Work out the finished part from the listing and answer in its coordinate system (mm). A direction names the side the tool comes from. Coordinates: 2 decimals unless noted, no trailing zeros. Loops run counter-clockwise (first coordinate to the right, second up) from the corner with the lowest first, then second, coordinate; pieces in that order, holes last. Notation, with made-up numbers: (-13, 39.25) -> (42, 39.25) arc R27 ccw to (42, 78.25) -> close; hole circle Ø8 at (51, 86.25). An arc over 180 degrees is marked (long way). Answer as CSV lines item,"result".
```python
from build123d import *

# Parameters (mm, degrees)
SKIZZE2_W                            = 100
SKIZZE2_H                            = 39.364160046
AUFSATZ_LINEAR_AUSTRAGEN1_DEPTH      = 30
SCHNITT_LINEAR_AUSTRAGEN1_DEPTH      = 40
SCHNITT_LINEAR_AUSTRAGEN1_DEPTH_BACK = 40
SKIZZE10_R                           = 5
SKIZZE17_R                           = 1.55
SCHNITT_LINEAR_AUSTRAGEN2_DEPTH      = 3
SKIZZE24_R                           = 1.55
SCHNITT_LINEAR_AUSTRAGEN4_DEPTH      = 112.577493681
SKIZZE37_R                           = 0.736865544
SCHNITT_LINEAR_AUSTRAGEN9_DEPTH      = 112.577493681
SKIZZE40_R                           = 2.1
SCHNITT_LINEAR_AUSTRAGEN10_DEPTH     = 6
SKIZZE42_R                           = 0.75
SCHNITT_LINEAR_AUSTRAGEN12_DEPTH     = 10
SKIZZE46_R                           = 2.85
SCHNITT_LINEAR_AUSTRAGEN15_DEPTH     = 10
SCHNITT_LINEAR_START                 = -5
SCHNITT_LINEAR_AUSTRAGEN25_DEPTH     = 2.7
LINEARES_MUSTER1_COUNT               = 5
LINEARES_MUSTER1_PITCH               = 17
SPIEGELN2_COPY_1_SKETCH_R            = 2.85
SPIEGELN2_COPY_1_DEPTH               = 10
SPIEGELN2_COPY_2_SKETCH_R            = 2.85
SPIEGELN2_COPY_2_DEPTH               = 10
SPIEGELN2_COPY_3_SKETCH_R            = 2.85
SPIEGELN2_COPY_3_DEPTH               = 10
SPIEGELN2_COPY_4_SKETCH_R            = 2.85
SPIEGELN2_COPY_4_DEPTH               = 10
SPIEGELN2_START                      = -5
SPIEGELN2_COPY_5_DEPTH               = 2.7
SPIEGELN2_COPY_6_DEPTH               = 2.7
SPIEGELN2_COPY_7_DEPTH               = 2.7
SPIEGELN2_COPY_8_DEPTH               = 2.7
SKIZZE51_R                           = 1.55
SCHNITT_LINEAR_AUSTRAGEN26_DEPTH     = 112.577493681
SKIZZE55_R                           = 0.5
SCHNITT_LINEAR_AUSTRAGEN28_DEPTH     = 112.577493681
SKIZZE59_R                           = 2.05
SCHNITT_LINEAR_AUSTRAGEN30_DEPTH     = 5
FASE1_SIZE                           = 1
FASE2_SIZE                           = 1
ABSPALTEN3_SURFACE_1_BACK            = 112.577
ABSPALTEN3_SURFACE_1_DEPTH           = 225.154


with BuildPart() as part:
    # Skizze2 → Aufsatz-Linear austragen1 (new body)
    with BuildSketch(Plane.XY):
        with Locations((50, 19.682080023)):
            Rectangle(SKIZZE2_W, SKIZZE2_H)
    extrude(amount=AUFSATZ_LINEAR_AUSTRAGEN1_DEPTH)

    # Skizze10 → Schnitt-Linear austragen1 (cut, two sides: drawn at the far end of the back side and taken through both)
    with BuildSketch(Plane.ZY.offset(-50).offset(-SCHNITT_LINEAR_AUSTRAGEN1_DEPTH_BACK)):
        with Locations((14.945770016, 20.027045739)):
            Circle(SKIZZE10_R)
    extrude(amount=SCHNITT_LINEAR_AUSTRAGEN1_DEPTH + SCHNITT_LINEAR_AUSTRAGEN1_DEPTH_BACK, mode=Mode.SUBTRACT)

    # Skizze17 → Schnitt-Linear austragen2 (cut)
    with BuildSketch(Plane.ZY.offset(-90)):
        with Locations((14.945770016, 20.027045739)):
            Circle(SKIZZE17_R)
    schnitt_linear_austragen2 = extrude(amount=-SCHNITT_LINEAR_AUSTRAGEN2_DEPTH, mode=Mode.SUBTRACT)

    # Spiegeln1: Schnitt-Linear austragen2 across plane
    add(schnitt_linear_austragen2.mirror(Plane.ZY.offset(-50)), mode=Mode.SUBTRACT)

    # Skizze24 → Schnitt-Linear austragen4 (cut, through all)
    with BuildSketch(Plane.XY.offset(30)):
        with Locations((16, 31.364160046)):
            Circle(SKIZZE24_R)
        with Locations((33, 31.364160046)):
            Circle(SKIZZE24_R)
        with Locations((50, 31.364160046)):
            Circle(SKIZZE24_R)
        with Locations((67, 31.364160046)):
            Circle(SKIZZE24_R)
        with Locations((84, 31.364160046)):
            Circle(SKIZZE24_R)
    schnitt_linear_austragen4 = extrude(amount=-SCHNITT_LINEAR_AUSTRAGEN4_DEPTH, mode=Mode.SUBTRACT)

    # Skizze37 → Schnitt-Linear austragen9 (cut, through all)
    with BuildSketch(Plane(origin=(100, 0, 0), x_dir=(0, 0, -1), z_dir=(1, 0, 0))):
        with Locations((-18.924590299, 18.633559666)):
            Circle(SKIZZE37_R)
    extrude(amount=-SCHNITT_LINEAR_AUSTRAGEN9_DEPTH, mode=Mode.SUBTRACT)

    # Skizze40 → Schnitt-Linear austragen10 (cut)
    with BuildSketch(Plane(origin=(100, 0, 0), x_dir=(0, 0, -1), z_dir=(1, 0, 0))):
        with Locations((-18.924590299, 18.633559666)):
            Circle(SKIZZE40_R)
    extrude(amount=-SCHNITT_LINEAR_AUSTRAGEN10_DEPTH, mode=Mode.SUBTRACT)

    # Skizze42 → Schnitt-Linear austragen12 (cut)
    with BuildSketch(Plane.ZY):
        with Locations((10.86415918, 18.842582577)):
            Circle(SKIZZE42_R)
    extrude(amount=-SCHNITT_LINEAR_AUSTRAGEN12_DEPTH, mode=Mode.SUBTRACT)

    # Skizze46 → Schnitt-Linear austragen15 (cut)
    with BuildSketch(Plane(origin=(0, 0, 0), x_dir=(-1, 0, 0), z_dir=(0, 0, -1))):
        with Locations((-84, 31.364160046)):
            Circle(SKIZZE46_R)
    schnitt_linear_austragen15 = extrude(amount=-SCHNITT_LINEAR_AUSTRAGEN15_DEPTH, mode=Mode.SUBTRACT)

    # Skizze50 → Schnitt-Linear austragen25 (cut)
    with BuildSketch(Plane.XY.offset(30).offset(SCHNITT_LINEAR_START)):
        Polygon((81.15, 33.009608314), (81.15, 39.364160046), (86.85, 39.364160046), (86.85, 33.009608314), (86.85, 29.718711779), (84, 28.073263512), (81.15, 29.718711779), align=None)
    schnitt_linear_austragen25 = extrude(amount=-SCHNITT_LINEAR_AUSTRAGEN25_DEPTH, mode=Mode.SUBTRACT)

    # Lineares Muster1: Schnitt-Linear austragen15, Schnitt-Linear austragen25 ×5
    with Locations(*[(-i * LINEARES_MUSTER1_PITCH, 0, 0) for i in range(1, LINEARES_MUSTER1_COUNT)]):
        add(schnitt_linear_austragen15, mode=Mode.SUBTRACT)
        add(schnitt_linear_austragen25, mode=Mode.SUBTRACT)

    # Spiegeln2: Schnitt-Linear austragen15, Schnitt-Linear austragen25 across plane
    add(schnitt_linear_austragen15.mirror(Plane.ZX.offset(19.764160046)), mode=Mode.SUBTRACT)
    add(schnitt_linear_austragen25.mirror(Plane.ZX.offset(19.764160046)), mode=Mode.SUBTRACT)

    # Spiegeln2 copy 1 sketch → Spiegeln2 copy 1 (cut)
    with BuildSketch(Plane(origin=(-17, 39.528320093, 0), x_dir=(-1, 0, 0), z_dir=(0, 0, -1))):
        with Locations((-84, -31.364160046)):
            Circle(SPIEGELN2_COPY_1_SKETCH_R)
    extrude(amount=-SPIEGELN2_COPY_1_DEPTH, mode=Mode.SUBTRACT)

    # Spiegeln2 copy 2 sketch → Spiegeln2 copy 2 (cut)
    with BuildSketch(Plane(origin=(-34, 39.528320093, 0), x_dir=(-1, 0, 0), z_dir=(0, 0, -1))):
        with Locations((-84, -31.364160046)):
            Circle(SPIEGELN2_COPY_2_SKETCH_R)
    extrude(amount=-SPIEGELN2_COPY_2_DEPTH, mode=Mode.SUBTRACT)

    # Spiegeln2 copy 3 sketch → Spiegeln2 copy 3 (cut)
    with BuildSketch(Plane(origin=(-51, 39.528320093, 0), x_dir=(-1, 0, 0), z_dir=(0, 0, -1))):
        with Locations((-84, -31.364160046)):
            Circle(SPIEGELN2_COPY_3_SKETCH_R)
    extrude(amount=-SPIEGELN2_COPY_3_DEPTH, mode=Mode.SUBTRACT)

    # Spiegeln2 copy 4 sketch → Spiegeln2 copy 4 (cut)
    with BuildSketch(Plane(origin=(-68, 39.528320093, 0), x_dir=(-1, 0, 0), z_dir=(0, 0, -1))):
        with Locations((-84, -31.364160046)):
            Circle(SPIEGELN2_COPY_4_SKETCH_R)
    extrude(amount=-SPIEGELN2_COPY_4_DEPTH, mode=Mode.SUBTRACT)

    # Spiegeln2 copy 5 sketch → Spiegeln2 copy 5 (cut)
    with BuildSketch(Plane(origin=(-17, 39.528320093, 30), x_dir=(1, 0, 0), z_dir=(0, 0, 1)).offset(SPIEGELN2_START)):
        Polygon((81.15, -33.009608314), (81.15, -39.364160046), (86.85, -39.364160046), (86.85, -33.009608314), (86.85, -29.718711779), (84, -28.073263512), (81.15, -29.718711779), align=None)
    extrude(amount=-SPIEGELN2_COPY_5_DEPTH, mode=Mode.SUBTRACT)

    # Spiegeln2 copy 6 sketch → Spiegeln2 copy 6 (cut)
    with BuildSketch(Plane(origin=(-34, 39.528320093, 30), x_dir=(1, 0, 0), z_dir=(0, 0, 1)).offset(SPIEGELN2_START)):
        Polygon((81.15, -33.009608314), (81.15, -39.364160046), (86.85, -39.364160046), (86.85, -33.009608314), (86.85, -29.718711779), (84, -28.073263512), (81.15, -29.718711779), align=None)
    extrude(amount=-SPIEGELN2_COPY_6_DEPTH, mode=Mode.SUBTRACT)

    # Spiegeln2 copy 7 sketch → Spiegeln2 copy 7 (cut)
    with BuildSketch(Plane(origin=(-51, 39.528320093, 30), x_dir=(1, 0, 0), z_dir=(0, 0, 1)).offset(SPIEGELN2_START)):
        Polygon((81.15, -33.009608314), (81.15, -39.364160046), (86.85, -39.364160046), (86.85, -33.009608314), (86.85, -29.718711779), (84, -28.073263512), (81.15, -29.718711779), align=None)
    extrude(amount=-SPIEGELN2_COPY_7_DEPTH, mode=Mode.SUBTRACT)

    # Spiegeln2 copy 8 sketch → Spiegeln2 copy 8 (cut)
    with BuildSketch(Plane(origin=(-68, 39.528320093, 30), x_dir=(1, 0, 0), z_dir=(0, 0, 1)).offset(SPIEGELN2_START)):
        Polygon((81.15, -33.009608314), (81.15, -39.364160046), (86.85, -39.364160046), (86.85, -33.009608314), (86.85, -29.718711779), (84, -28.073263512), (81.15, -29.718711779), align=None)
    extrude(amount=-SPIEGELN2_COPY_8_DEPTH, mode=Mode.SUBTRACT)

    # Spiegeln3: Schnitt-Linear austragen4 across plane
    add(schnitt_linear_austragen4.mirror(Plane.ZX.offset(19.764160046)), mode=Mode.SUBTRACT)

    # Skizze51 → Schnitt-Linear austragen26 (cut, through all)
    with BuildSketch(Plane.XY.offset(30)):
        with Locations((5, 34.364160046)):
            Circle(SKIZZE51_R)
        with Locations((95, 5)):
            Circle(SKIZZE51_R)
    extrude(amount=-SCHNITT_LINEAR_AUSTRAGEN26_DEPTH, mode=Mode.SUBTRACT)

    # Skizze55 → Schnitt-Linear austragen28 (cut, through all)
    with BuildSketch(Plane(origin=(100, 0, 0), x_dir=(0, 0, -1), z_dir=(1, 0, 0))):
        with Locations((-12.633679338, 21.083160509)):
            Circle(SKIZZE55_R)
    extrude(amount=-SCHNITT_LINEAR_AUSTRAGEN28_DEPTH, mode=Mode.SUBTRACT)

    # Skizze59 → Schnitt-Linear austragen30 (cut)
    with BuildSketch(Plane(origin=(100, 0, 0), x_dir=(0, 0, -1), z_dir=(1, 0, 0))):
        with Locations((-12.633679338, 21.083160509)):
            Circle(SKIZZE59_R)
    extrude(amount=-SCHNITT_LINEAR_AUSTRAGEN30_DEPTH, mode=Mode.SUBTRACT)

    # Fase1
    fase1_edges = [part.edges().sort_by_distance(p)[0] for p in [
        (94, 18.633559666, 19.661455843),
    ]]
    chamfer(fase1_edges, length=FASE1_SIZE)

    # Fase2
    fase2_edges = [part.edges().sort_by_distance(p)[0] for p in [
        (95, 21.083160509, 13.133679338),
    ]]
    chamfer(fase2_edges, length=FASE2_SIZE)

    # Abspalten3: cut with a surface, the side it looks to stays
    # Abspalten3 surface: a surface, the sketch's curves swept straight by 225.154 mm
    with BuildLine(Plane(origin=(100, 0, 0), x_dir=(0, 0, -1), z_dir=(1, 0, 0)).offset(-ABSPALTEN3_SURFACE_1_BACK), mode=Mode.PRIVATE) as abspalten3_surface_1_path:
        Line((-15, 39.364160046), (0, 39.364160046))
        Line((0, 39.364160046), (0, 0))
        Line((0, 0), (-15, 0))
        Line((-15, 0), (-15, 39.364160046))
    abspalten3_surface_1 = Shell.extrude(abspalten3_surface_1_path.wire(), (1 * ABSPALTEN3_SURFACE_1_DEPTH, 0 * ABSPALTEN3_SURFACE_1_DEPTH, 0 * ABSPALTEN3_SURFACE_1_DEPTH))
    split(bisect_by=abspalten3_surface_1, keep=Keep.TOP)


solid = part.part
```
(1) Flat-ended cylindrical pins translate along their axes: pin 1 Ø2.5 at (x, y) = (50, 31.36) entering from +Z; pin 2 Ø1.3 at (x, z) = (33, 23.5) entering from +Y; pin 3 Ø0.8 at (x, z) = (51.5, 24) entering from +Y; pin 4 Ø2 at (y, z) = (18.5, 18) entering from +X. Find the tip coordinate at first contact, or state that the pin passes through.
Computed values:
pin 1,"through"
pin 2,"y = 28.45"
pin 3,"y = 29.17"
pin 4,"x = 94"
(2) Consider line 1 along X through (y, z) = (8, 23.75); line 2 along Y through (x, z) = (16, 21.75); line 3 along X through (y, z) = (8, 25.75). Determine where each line is inside the solid, lowest interval first.
Computed values:
line 1,"0 to 13.15, 18.85 to 30.15, 35.85 to 47.15, 52.85 to 64.15, 69.85 to 81.15, 86.85 to 100"
line 2,"0 to 6.61, 9.71 to 29.81, 32.91 to 39.36"
line 3,"0 to 14.46, 17.54 to 31.46, 34.54 to 48.46, 51.54 to 65.46, 68.54 to 82.46, 85.54 to 100"
(3) A cutting plane is placed at A-A, the plane y = 5. Write down the section's boundary in (x, z).
Computed values:
outline,"(0, 15) -> (93.45, 15) -> (93.45, 30) -> (0, 30) -> close; (96.55, 15) -> (100, 15) -> (100, 30) -> (96.55, 30) -> close; hole (13.15, 22.3) -> (18.85, 22.3) -> (18.85, 25) -> (13.15, 25) -> close; hole (30.15, 22.3) -> (35.85, 22.3) -> (35.85, 25) -> (30.15, 25) -> close; hole (47.15, 22.3) -> (52.85, 22.3) -> (52.85, 25) -> (47.15, 25) -> close; hole (64.15, 22.3) -> (69.85, 22.3) -> (69.85, 25) -> (64.15, 25) -> close; hole (81.15, 22.3) -> (86.85, 22.3) -> (86.85, 25) -> (81.15, 25) -> close"
(4) A cutting plane is placed at D-D, the plane x = 5. Write down the section's boundary in (y, z).
Computed values:
outline,"(0, 15) -> (32.81, 15) -> (32.81, 30) -> (0, 30) -> close; (35.91, 15) -> (39.36, 15) -> (39.36, 30) -> (35.91, 30) -> close; hole circle Ø1.47 at (18.63, 18.92)"
(5) Which of the six approach directions +Z, -Z, +X, -X, +Y, -Y give full straight-line access (tool end or side, diameter ignored) to faces 5 (the face through (49, 0, 22)), 6 (the face through (65.595, 28.884, 23.669)), 7 (the face through (81.15, 5, 24))?
Computed values:
face 5,"+Z, -Z, +X, -X, -Y"
face 6,"+Y"
face 7,"none"
(6) For a pull along X with two mould halves and no side action, classify faces 1 (the face through (100, 19, 22)), 2 (the face through (97.042, 17.356, 20.591)), 3 (the face through (48.595, 28.884, 23.669)), 4 (the face through (0, 19, 22)) as pulls with the +X half, pulls with the -X half, needs draft (parallel to the pull), parting line crosses it, or undercut.
Computed values:
face 1,"pulls with the +X half"
face 2,"needs draft"
face 3,"undercut"
face 4,"pulls with the -X half"
(7) A cutting plane is placed at C-C, the plane z = 27.75. Count the separate pieces of the cut face and the enclosed holes in it, and give its area (3 significant figures).
Computed values:
separate pieces,"1"
enclosed holes,"12"
area,"3,850 mm2"
(8) A cutting plane is placed at B-B, the plane x = 95. Write down the section's boundary in (y, z).
Computed values:
outline,"(0, 15) -> (3.45, 15) -> (3.45, 30) -> (0, 30) -> close; (6.55, 15) -> (39.36, 15) -> (39.36, 30) -> (6.55, 30) -> close; hole circle Ø4.2 at (18.63, 18.92)"
